from build123d import *

# Parameters (mm, degrees)
F0_R     = 2
F1_DEPTH = 10
F2_SIZE  = 5
F3_R     = 5
F4_SIZE  = 1
F5_SIZE  = 0.5


with BuildPart() as f1:
    # F0 (on Top) → F1 (new body)
    with BuildSketch(Plane.XY):
        with BuildLine():
            Line((0, 20), (0, 0))
            Line((0, 0), (4, 0))
            Line((4, 0), (4, 10))
            Line((4, 10), (7.1, 10))
            Line((7.1, 10), (7.1, -15))
            Line((7.1, -15), (11.1, -15))
            Line((11.1, -15), (11.1, 10))
            Line((11.1, 10), (37.1, 10))
            ThreePointArc((37.1, 10), (42.1, 15), (37.1, 20))
            Line((37.1, 20), (0, 20))
        make_face()
        with Locations((37.1, 15)):
            Circle(F0_R, mode=Mode.SUBTRACT)
    extrude(amount=F1_DEPTH)

    # F2
    f2_edges = [f1.edges().sort_by_distance(p)[0] for p in [
        (0, 20, 5),
        (11.1, 10, 5),
    ]]
    chamfer(f2_edges, length=F2_SIZE)

    # F3
    f3_edges = [f1.edges().sort_by_distance(p)[0] for p in [
        (0, 15, 5),
        (5, 20, 5),
        (16.1, 10, 5),
        (11.1, 5, 5),
    ]]
    fillet(f3_edges, radius=F3_R)

    # F4
    f4_edges = [f1.edges().sort_by_distance(p)[0] for p in [
        (4, 0, 5),
        (7.1, -15, 5),
    ]]
    chamfer(f4_edges, length=F4_SIZE)

    # F5
    f5_edges = [f1.edges().sort_by_distance(p)[0] for p in [
        (0, 0, 5),
        (11.1, -15, 5),
        (27.635534, 10, 10),
        (27.635534, 10, 0),
        (1.5, 0, 10),
        (3.5, 0.5, 10),
        (4, 5.5, 10),
        (5.55, 10, 10),
        (7.1, -2, 10),
        (9.6, -15, 10),
        (7.6, -14.5, 10),
        (1.5, 0, 0),
        (3.5, 0.5, 0),
        (4, 5.5, 0),
        (5.55, 10, 0),
        (7.1, -2, 0),
        (7.6, -14.5, 0),
        (9.6, -15, 0),
    ]]
    chamfer(f5_edges, length=F5_SIZE)


solid = f1.part
Can you work these out from the model? Positions are in its coordinate system, mm. A direction names the side the tool comes from. Coordinates: 2 decimals unless noted, no trailing zeros. Loops run counter-clockwise (first coordinate to the right, second up) from the corner with the lowest first, then second, coordinate; pieces in that order, holes last. Notation, with made-up numbers: (-11.5, -1.5) - (34.5, -1.5) arc R26 cw to (34.5, 27.5) - close; hole circle Ø2 at (18.5, 42). An arc over 180 degrees is marked (long way). Put each result on its own line as item: value. Start each with the question number.
Item 1: Suppose I cut it at B-B (y = -7). Please give me the cut outline in (x, z), and give its area (3 significant figures).
Item 2: Suppose I cut it at A-A (z = 4). Please give me the cut outline in (x, y), and give its area (3 significant figures).
Item 3: Suppose I cut it at C-C (y = 7.5). Please give me the cut outline in (x, z), and give its area (3 significant figures).
Item 4: If we mould it in two halves opening along X, with no side actions, what happens to faces 3 (the face through (4, 5, 5)), 4 (the face through (16, 11, 10)), 5 (the face through (7.772, -14.314, 9.754))? For each: +X half, -X half, draft (parallel to the pull), parting line (faces both ways), or undercut.
Item 5: For pin 1 (5 mm diameter, centred on y = -10, z = 4, fed in from +X); pin 2 (5 mm diameter, centred on x = 4.5, z = 8, fed in from -Y); pin 3 (0.9 mm diameter, centred on x = 6, z = 7, fed in from -Y), each with a flat end and sliding along its axis, tell me the tip position at first contact or that it passes through.
Item 6: Suppose I cut it at D-D (x = 29). Please give me the cut outline in (y, z), and give its area (3 significant figures).
Item 7: Which directions (+Z, -Z, +X, -X, +Y, -Y) give clear straight access to the entire face, cutting with the end or side of a thin tool? Please do faces 1 (the face through (2.69, 17.34, 0.25)), 2 (the face through (3.5, 0.5, 4.9)).
Item 8: If I drill on line 1 along Y through (x, z) = (37.1, 4); line 2 along X through (y, z) = (-9, 2.25); line 3 along X through (y, z) = (16.5, 8.75), over which ranges is the centre line in solid material (lowest first)?
Here are the results:
1. outline: (7.1, 0.5) - (7.6, 0) - (10.6, 0) - (11.1, 0.5) - (11.1, 9.5) - (10.6, 10) - (7.6, 10) - (7.1, 9.5) - close
1. area: 39.5 mm²
2. outline: (0, 0.5) - (0.5, 0) - (3, 0) - (4, 1) - (4, 10) - (7.1, 10) - (7.1, -14) - (8.1, -15) - (10.6, -15) - (11.1, -14.5) - (11.1, 2.93) arc R5 cw to (12.56, 6.46) - (14.64, 8.54) arc R5 cw to (18.17, 10) - (37.1, 10) arc R5 ccw to (37.1, 20) - (7.07, 20) arc R5 ccw to (3.54, 18.54) - (1.46, 16.46) arc R5 ccw to (0, 12.93) - close; hole circle Ø4 at (37.1, 15)
2. area: 536 mm²
3. outline: (0, 0.5) - (0.5, 0) - (3.5, 0) - (4, 0.5) - (4, 9.5) - (3.5, 10) - (0.5, 10) - (0, 9.5) - close; (7.1, 0.5) - (7.6, 0) - (12.89, 0) - (13.6, 0.5) - (13.6, 9.5) - (12.89, 10) - (7.6, 10) - (7.1, 9.5) - close
3. area: 104 mm²
4. face 3: undercut
4. face 4: draft
4. face 5: -X half
5. pin 1: x = 11.1
5. pin 2: y = 0
5. pin 3: y = 10
6. outline: (10, 0.5) - (10.5, 0) - (19.5, 0) - (20, 0.5) - (20, 9.5) - (19.5, 10) - (10.5, 10) - (10, 9.5) - close
6. area: 99.5 mm²
7. face 1: -Z, -X, +Y
7. face 2: +Z, -Z, -Y
8. line 1: 10 to 13, 17 to 20
8. line 2: 7.1 to 11.1
8. line 3: 1.5 to 35.78, 38.42 to 41.87
